Check sheet for the modelled part. Datum: model origin and axes. Units: mm. A direction names the side the tool comes from. Give positions to 0.01 mm unless a question says otherwise; leave off trailing zeros. Order: outer loops, then holes, each group sorted by start corner. A loop starts at its lowest first (then second) coordinate and runs counter-clockwise, first axis right, second up.
from build123d import *

# Parameters (mm, degrees)
BOSS_EXTRUDE1_DEPTH       = 7.5
SKETCH2_R                 = 3.587141307
BOSS_EXTRUDE2_DEPTH       = 4.3
F_4_CLEARANCE_HOLE1_D     = 3.2639
F_4_CLEARANCE_HOLE1_DEPTH = 5.84
F_4_CLEARANCE_HOLE1_TIP   = 0.980574487


with BuildPart() as part:
    # Sketch1 → Boss-Extrude1 (new, symmetric)
    with BuildSketch(Plane.XY):
        Polygon((-14.75, 11.925), (-20, 11.925), (-20, 13.925), (-14.75, 13.925), (-14.75, 18.474377385), (-11.75, 20.575), (13.27912821, 20.575), (14.75, 18.474377385), (14.75, 13.925), (20, 13.925), (20, 11.925), (14.75, 11.925), (14.75, -11.925), (-14.75, -11.925), align=None)
    extrude(amount=BOSS_EXTRUDE1_DEPTH, both=True)

    # Sketch2 → Boss-Extrude2 (add)
    with BuildSketch(Plane(origin=(0, 20.575, 0), x_dir=(1, 0, 0), z_dir=(0, 1, 0))):
        with Locations((7.375, 0)):
            Circle(SKETCH2_R)
    extrude(amount=BOSS_EXTRUDE2_DEPTH)

    # #4 Clearance Hole1
    with Locations(Plane(origin=(0, 13.925, 0), x_dir=(1, 0, 0), z_dir=(0, 1, 0))):
        with Locations((-17.65, 0), (17.65, 0)):
            Hole(F_4_CLEARANCE_HOLE1_D / 2, depth=F_4_CLEARANCE_HOLE1_DEPTH)
            with Locations((0, 0, -(F_4_CLEARANCE_HOLE1_DEPTH + F_4_CLEARANCE_HOLE1_TIP / 2))):  # 118° drill point
                Cone(0, F_4_CLEARANCE_HOLE1_D / 2, F_4_CLEARANCE_HOLE1_TIP, mode=Mode.SUBTRACT)


solid = part.part
1) Section check C-C, the plane z = -5. Record the cut outline in (x, y) (3 decimals), then the cut area to 3 significant figures.
Recorded:
outline: (-20, 11.925) - (-14.75, 11.925) - (-14.75, -11.925) - (14.75, -11.925) - (14.75, 11.925) - (20, 11.925) - (20, 13.925) - (14.75, 13.925) - (14.75, 18.474) - (13.279, 20.575) - (-11.75, 20.575) - (-14.75, 18.474) - (-14.75, 13.925) - (-20, 13.925) - close
area: 975 mm2
2) Set-up check for faces 4 (the face through (-14.75, 0, 0)), 5 (the face through (-14.75, 16, 0)), 6 (the face through (17, 11.925, 2)), 7 (the face through (19.28, 12.91, -0.07)), 8 (the face through (17, 13.925, 2)): record each of +Z, -Z, +X, -X, +Y, -Y from which the full face is reachable in a straight line by a thin tool's end or side.
Recorded:
face 4: +Z, -Z, -X, -Y
face 5: +Z, -Z, -X, +Y
face 6: +Z, -Z, +X, -Y
face 7: +Y, -Y
face 8: +Z, -Z, +X, +Y
3) Material ranges on L1, parallel to Z at x = 17.65, y = 12.6; L2, parallel to Y at x = -11.5, z = 1 (3 decimals); L3, parallel to X at y = 11, z = 3.75, recorded low to high.
Recorded:
L1: z = -7.5 to -1.63, 1.63 to 7.5
L2: y = -11.925 to 20.575
L3: x = -14.75 to 14.75
4) Section check B-B, the plane x = -17.65. Record the cut outline in (y, z) (3 decimals), then the cut area to 3 significant figures.
Recorded:
outline: (11.925, -7.5) - (13.925, -7.5) - (13.925, -1.632) - (11.925, -1.632) - close; (11.925, 1.632) - (13.925, 1.632) - (13.925, 7.5) - (11.925, 7.5) - close
area: 23.5 mm2
5) Depth check by flat-ended pin: pin 1 Ø1.5 at (y, z) = (15.5, -5.5) entering from +X; pin 2 Ø2.5 at (x, z) = (-17, -2.5) entering from +Y (3 decimals); pin 3 Ø4 at (x, z) = (17.65, 0) entering from -Y (3 decimals); pin 4 Ø5 at (y, z) = (15.5, 1) entering from +X. Enter the tip coordinate at first touch or a pass-through.
Recorded:
pin 1: stops at x = 14.75
pin 2: stops at y = 13.925
pin 3: stops at y = 11.925
pin 4: stops at x = 20
6) Section check D-D, the plane y = 15. Record the cut outline in (x, z), then the cut area to 4 significant figures.
Recorded:
outline: (-14.75, -7.5) - (14.75, -7.5) - (14.75, 7.5) - (-14.75, 7.5) - close
area: 442.5 mm2
7) Section check A-A, the plane z = 0. Record the cut outline in (x, y) (3 decimals), then the cut area to 3 significant figures.
Recorded:
outline: (-20, 11.925) - (-19.282, 11.925) - (-19.282, 13.925) - (-20, 13.925) - close; (-16.018, 11.925) - (-14.75, 11.925) - (-14.75, -11.925) - (14.75, -11.925) - (14.75, 11.925) - (16.018, 11.925) - (16.018, 13.925) - (14.75, 13.925) - (14.75, 18.474) - (13.279, 20.575) - (10.962, 20.575) - (10.962, 24.875) - (3.788, 24.875) - (3.788, 20.575) - (-11.75, 20.575) - (-14.75, 18.474) - (-14.75, 13.925) - (-16.018, 13.925) - close; (19.282, 11.925) - (20, 11.925) - (20, 13.925) - (19.282, 13.925) - close
area: 993 mm2
8) Draft check along X on faces 1 (the face through (-17, 11.925, 2)), 2 (the face through (-20, 13, 0)), 3 (the face through (-19.207, 12.911, -0.49)). Enter one of: +X half, -X half, draft (parallel to the pull), parting line (faces both ways), or undercut.
Recorded:
face 1: draft
face 2: -X half
face 3: undercut
